Part model, mm, in its own coordinate system. A direction names the side the tool comes from. Round coordinates to 2 decimals unless told otherwise and drop trailing zeros. Write each loop counter-clockwise with the first axis right and the second up, starting at its lowest first coordinate (ties: lowest second). Pieces come first, ordered by that corner, then holes.
Autodesk Inventor part; units mm, degrees
ref_plane "Plano de trabalho1" through (0, 39.4, 0) normal (0, 1, 0) x (-1, 0, 0)
ref_plane "YZ Plane" through (0, 0, 0) normal (1, 0, 0) x (0, 1, 0)
ref_plane "XY Plane" through (0, 0, 0) normal (0, 0, 1) x (1, 0, 0)
sketch "Esboço1" plane through (0, 0, 0) normal (0, 1, 0) x (-1, 0, 0)
  line L0 (-49, 49) -> (49, 49)
  line L1 (49, 49) -> (49, -49)
  line L2 (49, -49) -> (-49, -49)
  line L3 (-49, -49) -> (-49, 49)
  line L4 (-49, 49) -> (49, -49) construction
  line L5 (49, 49) -> (-49, -49) construction
  point P0 (0, 0)
  dimension "d0" = 98
  dimension "d1" = 98
extrude "Extrusão1" add sketch "Esboço1" along normal blind 39.4
shell "Casca1" thickness 2 removed faces 1 at (16.3333, 39.4, 16.3333)
sketch "Esboço3" plane through (0, 0, 0) normal (0, 0, 1) x (1, 0, 0)
  line L0 (0, 0) -> (32, 0)
  line L1 (49, 0) -> (-49, 0)
  line L2 (32, 0) -> (0, 36.5533)
  line L3 (0, 0) -> (0, 36.5533)
  point P0 (-43.1, 0)
  dimension "d6" = 32
  dimension "d7" = 48.8
revolve "Revolução1" add sketch "Esboço3" angle 360 about axis through (0, 0, 0) along (0, 1, 0)
sketch "Esboço4" plane through (0, 0, 0) normal (0, 0, 1) x (1, 0, 0)
  line L0 (0, 0) -> (30, 0)
  line L1 (-49, 0) -> (49, 0)
  line L2 (0, 36.5533) -> (-30.2491, 2)
  line L3 (30, 0) -> (0, 34.2687)
  line L4 (0, 0) -> (0, 34.2687)
  point P0 (43.1, 0)
  dimension "d9" = 30
  dimension "d10" = 48.8
revolve "Revolução2" cut sketch "Esboço4" angle 360 about axis through (0, 0, 0) along (0, 1, 0)
ref_plane "Plano de trabalho1" through (0, 39.4, 0) normal (0, 1, 0) x (-1, 0, 0)
sketch "Esboço5" plane through (0, 39.4, 0) normal (0, 1, 0) x (-1, 0, 0)
  line L0 (31.6566, 29.5617) -> (-31.6566, 29.5617)
  line L1 (-31.6566, 29.5617) -> (-31.6566, -29.5617)
  line L2 (-31.6566, -29.5617) -> (31.6566, -29.5617)
  line L3 (31.6566, -29.5617) -> (31.6566, 29.5617)
  line L4 (31.6566, 29.5617) -> (-31.6566, -29.5617) construction
  line L5 (-31.6566, 29.5617) -> (31.6566, -29.5617) construction
  point P0 (0, 0)
extrude "Extrusão2" cut sketch "Esboço5" against normal blind 18.8
sketch "Esboço6" plane through (0, 0, 0) normal (0, 1, 0) x (-1, 0, 0)
  point P0 (0, 0)
fillet "Arredondamento2" radius 2 8 edges at (47, 20.7, 47) (49, 19.7, 49) (-47, 20.7, 47) (-49, 19.7, 49) (-49, 19.7, -49) (-47, 20.7, -47) (49, 19.7, -49) (47, 20.7, -47)
properties part number "contenção"
Q1. Saw through at B-B, the plane z = 38. Write the cut outline in (x, y), and give its area (3 significant figures).
Q2. Saw through at A-A, the plane y = 12. Write the cut outline in (x, z), and give its area (3 significant figures).
Q3. Wall check: line 1 (X direction, y = 29, z = 22); line 2 (X direction, y = 19, z = -9). Give the ranges that are in metal, low to high.
Q4. Saw through at C-C, the plane y = 36. Write the cut outline in (x, z), and give its area (3 significant figures).
Q5. Tool access for faces 1 (the flat face through (-47, 20, 1)), 2 (the flat face through (49, 19, -1)): list every direction of +Z, -Z, +X, -X, +Y, -Y with a clear straight run to the whole face (end or side of a thin tool).
Q6. Saw through at D-D, the plane x = 0. Write the cut outline in (y, z).
Q7. Drop a flat-ended pin along its axis: P1, Ø10, axis at x = -16, z = 4, coming from the +Y side. Give the stop position or say it passes through.
Computed:
1. outline: (-49, 0) - (49, 0) - (49, 39.4) - (47, 39.4) - (47, 2) - (-47, 2) - (-47, 39.4) - (-49, 39.4) - close
1. area: 346 mm2
2. outline: (-49, -47) arc R2 ccw to (-47, -49) - (47, -49) arc R2 ccw to (49, -47) - (49, 47) arc R2 ccw to (47, 49) - (-47, 49) arc R2 ccw to (-49, 47) - close; circle Ø42.99 at (0, 0); hole (-47, -45) arc R2 ccw to (-45, -47) - (45, -47) arc R2 ccw to (47, -45) - (47, 45) arc R2 ccw to (45, 47) - (-45, 47) arc R2 ccw to (-47, 45) - close; hole circle Ø38.99 at (0, 0)
2. area: 1,030 mm2
3. line 1: x = -49 to -47, 47 to 49
3. line 2: x = -49 to -47, -12.46 to -9.88, 9.88 to 12.46, 47 to 49
4. outline: (-49, -47) arc R2 ccw to (-47, -49) - (47, -49) arc R2 ccw to (49, -47) - (49, 47) arc R2 ccw to (47, 49) - (-47, 49) arc R2 ccw to (-49, 47) - close; hole (-47, -45) arc R2 ccw to (-45, -47) - (45, -47) arc R2 ccw to (47, -45) - (47, 45) arc R2 ccw to (45, 47) - (-45, 47) arc R2 ccw to (-47, 45) - close
4. area: 768 mm2
5. face 1: +Y
5. face 2: +Z, -Z, +X, +Y, -Y
6. outline: (0, -49) - (39.4, -49) - (39.4, -47) - (2, -47) - (2, -30.25) - (20.6, -13.97) - (20.6, -11.97) - (0, -30) - close; (0, 30) - (20.6, 11.97) - (20.6, 13.97) - (2, 30.25) - (2, 47) - (39.4, 47) - (39.4, 49) - (0, 49) - close
7. P1: stops at y = 20.6
